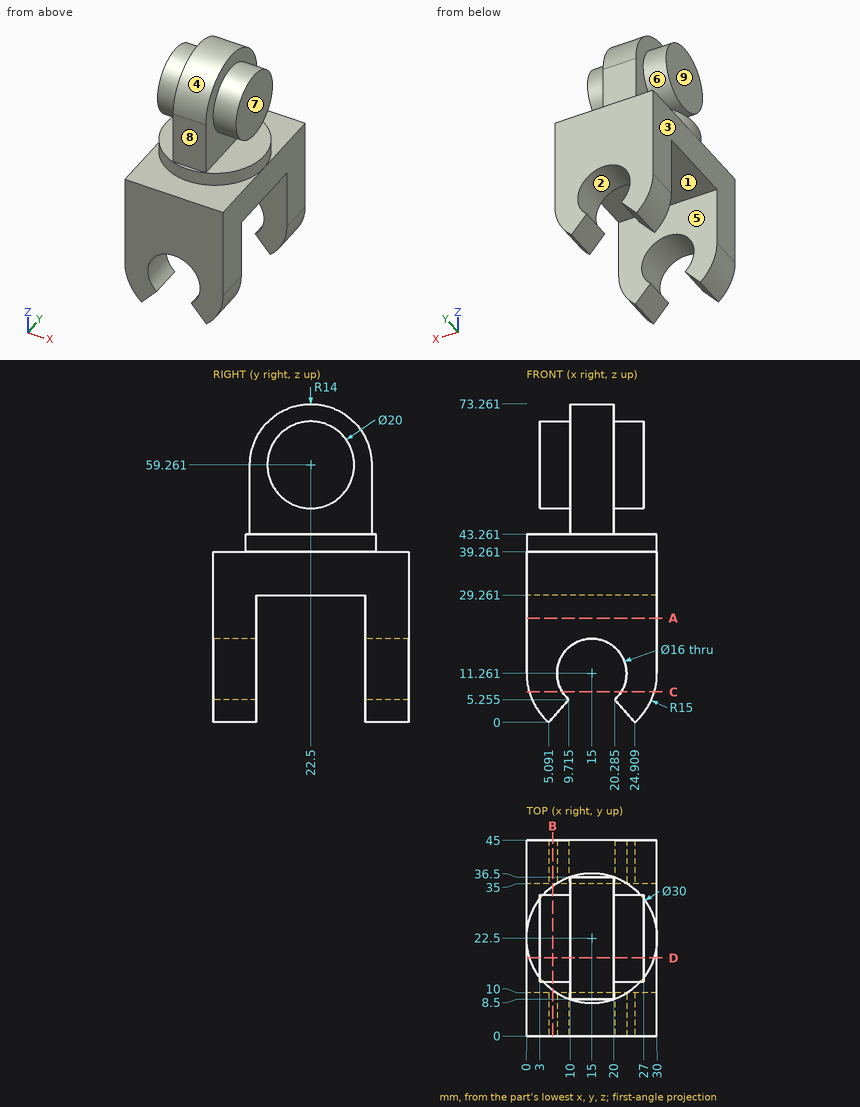
Can you work these out from the drawing? Everything is in mm from the part's minimum corner. A direction names the side the tool comes from. Coordinates: 2 decimals unless noted, no trailing zeros. Loops run counter-clockwise (first coordinate to the right, second up) from the corner with the lowest first, then second, coordinate; pieces in that order, holes last. Notation, with made-up numbers: (-19, 11.5) - (-14, 11.5) arc R22 ccw to (-14, 27.5) - close; hole circle Ø2 at (13.5, 68.25). An arc over 180 degrees is marked (long way). Answer as CSV lines item,"result".
Q1. If we section it at D-D, the plane y = 18: Write out the boundary of the cut face in (x, z), and give its area (3 significant figures).
Response:
outline,"(0, 29.26) - (30, 29.26) - (30, 39.26) - (29.31, 39.26) - (29.31, 43.26) - (20, 43.26) - (20, 50.33) - (27, 50.33) - (27, 68.19) - (20, 68.19) - (20, 72.52) - (10, 72.52) - (10, 68.19) - (3, 68.19) - (3, 50.33) - (10, 50.33) - (10, 43.26) - (0.69, 43.26) - (0.69, 39.26) - (0, 39.26) - close"
area,"957 mm2"
Q2. If we section it at A-A, the plane z = 24: Write out the boundary of the cut face in (x, y), and give its area (3 significant figures).
Response:
outline,"(0, 0) - (30, 0) - (30, 10) - (0, 10) - close; (0, 35) - (30, 35) - (30, 45) - (0, 45) - close"
area,"600 mm2"
Q3. We'd pull the mould along Z, two halves only. Please class the marked faces 1, 2, 3 and 4: pulls with the +Z half, pulls with the -Z half, needs draft (parallel to the pull), parting line crosses it, or undercut.
Response:
face 1,"pulls with the -Z half"
face 2,"undercut"
face 3,"needs draft"
face 4,"pulls with the +Z half"
Q4. If I drill on L1, parallel to Y at x = 8.75, z = 20; L2, parallel to Z at x = 15, y = 40.5; L3, parallel to Z at x = 8, y = 8.5 (1 decimal), over which ranges is the centre line in solid material (lowest first)? Write a range as [from, to].
Response:
L1,"[0, 10], [35, 45]"
L2,"[19.26, 39.26]"
L3,"[3.3, 7.4], [15.1, 39.3]"
Q5. If we section it at C-C, the plane z = 7: Write out the boundary of the cut face in (x, y).
Response:
outline,"(0.62, 0) - (8.23, 0) - (8.23, 10) - (0.62, 10) - close; (0.62, 35) - (8.23, 35) - (8.23, 45) - (0.62, 45) - close; (21.77, 0) - (29.38, 0) - (29.38, 10) - (21.77, 10) - close; (21.77, 35) - (29.38, 35) - (29.38, 45) - (21.77, 45) - close"
Q6. For pin 1 (6 mm diameter, centred on y = 20.5, z = 62.5, fed in from -X); pin 2 (1.5 mm diameter, centred on x = 20, y = 35, fed in from +Z); pin 3 (1.5 mm diameter, centred on y = 11.5, z = 48, fed in from +X), each with a flat end and sliding along its axis, tell me the tip position at first contact or that it passes through.
Response:
pin 1,"x = 3"
pin 2,"z = 66.87"
pin 3,"x = 20"
Q7. For the marked faces 5, 6, 7, 8 and 9, which set-ups out of +Z, -Z, +X, -X, +Y, -Y let a thin tool reach every point of the face, with its end or its side?
Response:
face 5,"-Z, +X, -X"
face 6,"-X"
face 7,"+Z, +X, +Y, -Y"
face 8,"+Z, +X, -X, -Y"
face 9,"+Z, -X, +Y, -Y"
Q8. If we section it at B-B, the plane x = 6: Write out the boundary of the cut face in (y, z), and give its area (3 significant figures).
Response:
outline,"(0, 1.03) - (10, 1.03) - (10, 29.26) - (35, 29.26) - (35, 1.03) - (45, 1.03) - (45, 39.26) - (34.5, 39.26) - (34.5, 43.26) - (10.5, 43.26) - (10.5, 39.26) - (0, 39.26) - close; circle Ø20 at (22.5, 59.26)"
area,"1,420 mm2"
